Check sheet for the drawn part. Datum: minimum x, y, z corner. Units: mm. Coordinates: 2 decimals unless noted, no trailing zeros. Order: outer loops, then holes, each group sorted by start corner. A loop starts at its lowest first (then second) coordinate and runs counter-clockwise, first axis right, second up.
1. Gauge pin test, flat ends, axial feed: pin 1 Ø2 at (y, z) = (19, 6) entering from +X; pin 2 Ø2 at (x, z) = (31, 4.5) entering from -Y; pin 3 Ø2 at (y, z) = (63, 3.5) entering from +X. Record the tip position at first contact, or that the pin passes through.
2. Cross-section at A-A (x = 50). Enter the section's corners in (y, z).
3. Draft check along Y on the marked faces 1, 2, 3 and 4. Enter one of: released by +Y, released by -Y, zero draft, split by the parting line, or undercut.
4. Cross-section at D-D (z = 1.5). Enter the section's corners in (x, y), then the cut area to 3 significant figures.
5. Cross-section at C-C (y = 80.5). Enter the section's corners in (x, z).
6. Thickness scan on line 1 (X direction, y = 51, z = 8.75); line 2 (Z direction, x = 6, y = 49); line 3 (Y direction, x = 50, z = 6). Record the ranges inside material, lowest first.
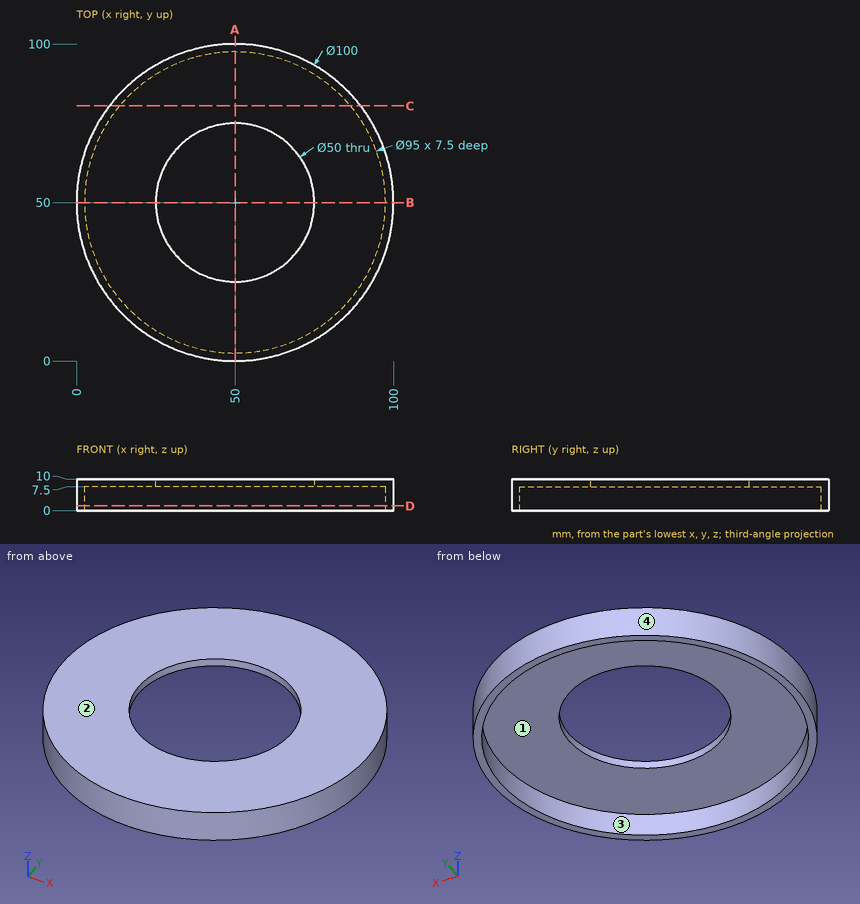
Data:
1. pin 1: stops at x = 90
1. pin 2: stops at y = 3.35
1. pin 3: stops at x = 98.54
2. outline: (0, 0) - (2.5, 0) - (2.5, 7.5) - (25, 7.5) - (25, 10) - (0, 10) - close; (75, 7.5) - (97.5, 7.5) - (97.5, 0) - (100, 0) - (100, 10) - (75, 10) - close
3. face 1: undercut
3. face 2: zero draft
3. face 3: undercut
3. face 4: split by the parting line
4. outline: circle Ø100 at (50, 50); hole circle Ø95 at (50, 50)
4. area: 766 mm2
5. outline: (10.38, 0) - (13.59, 0) - (13.59, 7.5) - (86.41, 7.5) - (86.41, 0) - (89.62, 0) - (89.62, 10) - (10.38, 10) - close
6. line 1: x = 0.01 to 25.02, 74.98 to 99.99
6. line 2: z = 7.5 to 10
6. line 3: y = 0 to 2.5, 97.5 to 100
